Verification items for this drawing (mm, ordinates from the low corner). Round coordinates to 2 decimals unless told otherwise and drop trailing zeros. Loops run counter-clockwise (first coordinate to the right, second up) from the corner with the lowest first, then second, coordinate; pieces in that order, holes last. Notation, with made-up numbers: M 70,-6 L 129,-6 A20 cw 129,20 Z; hole C 42.5,11 d11. An arc over 180 degrees is marked long. Write item = value, one per line.
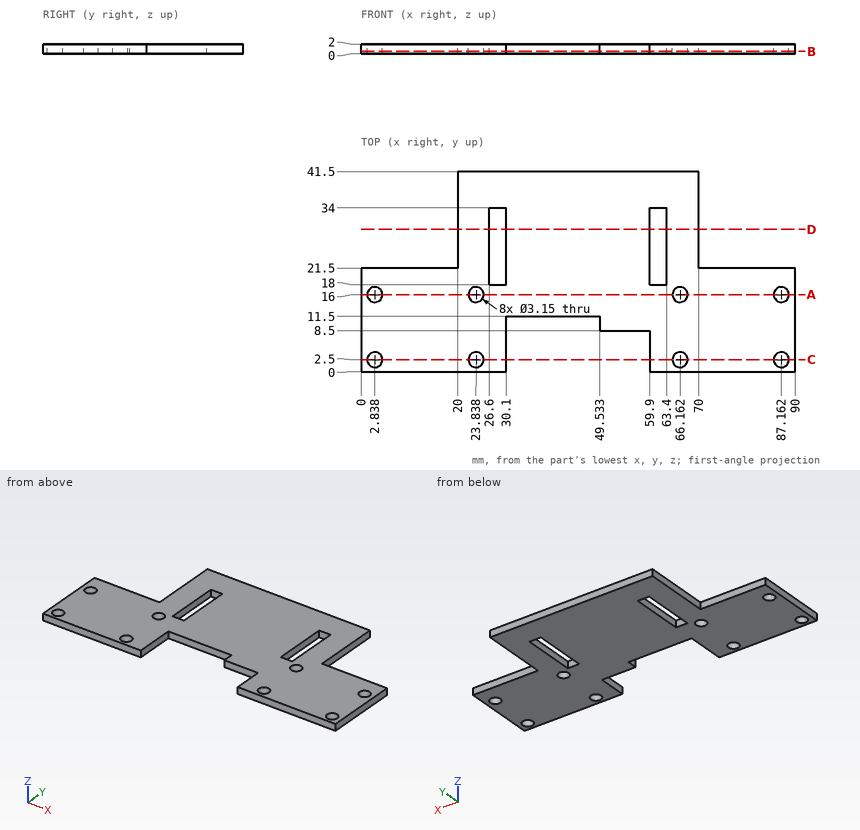
(1) Sectioned sample at A-A on y = 16. Record the cut outline in (x, z).
Result set:
outline = M 0,0 L 1.26,0 L 1.26,2 L 0,2 Z; M 4.41,0 L 22.26,0 L 22.26,2 L 4.41,2 Z; M 25.41,0 L 64.59,0 L 64.59,2 L 25.41,2 Z; M 67.74,0 L 85.59,0 L 85.59,2 L 67.74,2 Z; M 88.74,0 L 90,0 L 90,2 L 88.74,2 Z
(2) Material ranges on line 1 along X through (y, z) = (24, 1.6); line 2 along X through (y, z) = (16, 1.6); line 3 along X through (y, z) = (4.5, 1.65), recorded low to high. Write a range as from..to.
Result set:
line_1 = 20..26.6, 30.1..59.9, 63.4..70
line_2 = 0..1.26, 4.41..22.26, 25.41..64.59, 67.74..85.59, 88.74..90
line_3 = 0..30.1, 59.9..90
(3) Sectioned sample at B-B on z = 0.45. State how many separate pieces and enclosed holes the cut face has, then the cut area to 3 significant figures.
Result set:
separate_pieces = 1
enclosed_holes = 10
area = 2,450 mm2
(4) Sectioned sample at D-D on y = 29.5. Record the cut outline in (x, z).
Result set:
outline = M 20,0 L 26.6,0 L 26.6,2 L 20,2 Z; M 30.1,0 L 59.9,0 L 59.9,2 L 30.1,2 Z; M 63.4,0 L 70,0 L 70,2 L 63.4,2 Z
(5) Depth check by flat-ended pin: pin 1 Ø4 at (x, y) = (2.84, 2.5) entering from -Z; pin 2 Ø0.6 at (x, z) = (54, 1.5) entering from -Y; pin 3 Ø0.6 at (y, z) = (33, 1) entering from -X; pin 4 Ø1 at (y, z) = (25.5, 1.5) entering from +X. Enter the tip coordinate at first touch or a pass-through.
Result set:
pin_1 = 0
pin_2 = 8.5
pin_3 = 20
pin_4 = 70
(6) Sectioned sample at C-C on y = 2.5. Record the cut outline in (x, z).
Result set:
outline = M 0,0 L 1.26,0 L 1.26,2 L 0,2 Z; M 4.41,0 L 22.26,0 L 22.26,2 L 4.41,2 Z; M 25.41,0 L 30.1,0 L 30.1,2 L 25.41,2 Z; M 59.9,0 L 64.59,0 L 64.59,2 L 59.9,2 Z; M 67.74,0 L 85.59,0 L 85.59,2 L 67.74,2 Z; M 88.74,0 L 90,0 L 90,2 L 88.74,2 Z
